Could you check a few things on this model? Use its own coordinates, in mm. A direction names the side the tool comes from. Round coordinates to 2 decimals unless told otherwise and drop trailing zeros. Write each loop counter-clockwise with the first axis right and the second up, starting at its lowest first coordinate (ties: lowest second). Pieces come first, ordered by that corner, then holes.
```python
from build123d import *

# Parameters (mm, degrees)
F0_R      = 37.5
F1_DEPTH  = 1
F2_R      = 36
F3_DEPTH  = 4
F4_R      = 37.5
F4_R_2    = 36
F5_DEPTH  = 1
F7_DEPTH  = 6
F8_DEPTH  = 1
F9_R      = 2.5
F10_DEPTH = 20


with BuildPart() as f1:
    # F0 (on Front) → F1 (new body)
    with BuildSketch(Plane.XZ):
        Circle(F0_R)
    extrude(amount=F1_DEPTH)

    # F2 (on face) → F3 (join)
    with BuildSketch(Plane.XZ.offset(1)):
        Circle(F2_R)
    extrude(amount=F3_DEPTH)

    # F4 (on face) → F5 (join)
    with BuildSketch(Plane.XZ.offset(5)):
        Circle(F4_R)
        Circle(F4_R_2, mode=Mode.SUBTRACT)
    extrude(amount=F5_DEPTH)

    # F6 (on face) → F7 (join)
    with BuildSketch(Plane.XZ.offset(5)):
        with BuildLine():
            ThreePointArc((-14.3973607657, 4.3698820625), (-13.2562102609, 2.7015956993), (-14.8554257168, 1.4655075997))
            ThreePointArc((-14.8554257168, 1.4655075997), (-16.4714294815, 0.0592412802), (-14.9737084003, -1.4723868378))
            ThreePointArc((-14.9737084003, -1.4723868378), (-13.2809972538, -2.5769830711), (-14.2854492449, -4.3309728264))
            ThreePointArc((-14.2854492449, -4.3309728264), (-15.2402872256, -6.2486113636), (-13.270444668, -7.0904981892))
            ThreePointArc((-13.270444668, -7.0904981892), (-13.2509857133, -7.078215185), (-13.2313372043, -7.0662377391))
            ThreePointArc((-13.2313372043, -7.0662377391), (-11.2704807141, -7.4819524915), (-11.5406426234, -9.4681019001))
            ThreePointArc((-11.5406426234, -9.4681019001), (-11.5683788085, -9.4914339833), (-11.5955323776, -9.515441602))
            ThreePointArc((-11.5955323776, -9.515441602), (-11.6640462748, -11.6315042777), (-9.5468760318, -11.6291454669))
            ThreePointArc((-9.5468760318, -11.6291454669), (-9.5335988041, -11.6103508311), (-9.5200295189, -11.5917659551))
            ThreePointArc((-9.5200295189, -11.5917659551), (-7.5493471931, -11.2254490142), (-7.0388777787, -13.163798288))
            ThreePointArc((-7.0388777787, -13.163798288), (-6.3580749762, -15.1949459127), (-4.3698820625, -14.3973607657))
            ThreePointArc((-4.3698820625, -14.3973607657), (-2.7015956993, -13.2562102609), (-1.4655075997, -14.8554257168))
            ThreePointArc((-1.4655075997, -14.8554257168), (-0.0592412802, -16.4714294815), (1.4723868378, -14.9737084003))
            ThreePointArc((1.4723868378, -14.9737084003), (2.5769830711, -13.2809972538), (4.3309728264, -14.2854492449))
            ThreePointArc((4.3309728264, -14.2854492449), (6.2486113636, -15.2402872256), (7.0904981892, -13.270444668))
            ThreePointArc((7.0904981892, -13.270444668), (7.4632395293, -11.2838728073), (9.4681019001, -11.5406426234))
            ThreePointArc((9.4681019001, -11.5406426234), (11.6051695712, -11.6889493932), (11.6291454669, -9.5468760318))
            ThreePointArc((11.6291454669, -9.5468760318), (11.2132854236, -7.5688810145), (13.163798288, -7.0388777787))
            ThreePointArc((13.163798288, -7.0388777787), (15.1949459127, -6.3580749762), (14.3973607657, -4.3698820625))
            ThreePointArc((14.3973607657, -4.3698820625), (13.2562102609, -2.7015956993), (14.8554257168, -1.4655075997))
            ThreePointArc((14.8554257168, -1.4655075997), (16.4714294815, -0.0592412802), (14.9737084003, 1.4723868378))
            ThreePointArc((14.9737084003, 1.4723868378), (13.2809972538, 2.5769830711), (14.2854492449, 4.3309728264))
            ThreePointArc((14.2854492449, 4.3309728264), (15.2402872256, 6.2486113636), (13.270444668, 7.0904981892))
            ThreePointArc((13.270444668, 7.0904981892), (11.2838728073, 7.4632395293), (11.5406426234, 9.4681019001))
            ThreePointArc((11.5406426234, 9.4681019001), (11.6889493932, 11.6051695712), (9.5468760318, 11.6291454669))
            ThreePointArc((9.5468760318, 11.6291454669), (7.5688810145, 11.2132854236), (7.0388777787, 13.163798288))
            ThreePointArc((7.0388777787, 13.163798288), (6.3580749762, 15.1949459127), (4.3698820625, 14.3973607657))
            ThreePointArc((4.3698820625, 14.3973607657), (2.7015956993, 13.2562102609), (1.4655075997, 14.8554257168))
            ThreePointArc((1.4655075997, 14.8554257168), (0.0592412802, 16.4714294815), (-1.4723868378, 14.9737084003))
            ThreePointArc((-1.4723868378, 14.9737084003), (-2.5769830711, 13.2809972538), (-4.3309728264, 14.2854492449))
            ThreePointArc((-4.3309728264, 14.2854492449), (-6.2486113636, 15.2402872256), (-7.0904981892, 13.270444668))
            ThreePointArc((-7.0904981892, 13.270444668), (-7.4632395293, 11.2838728073), (-9.4681019001, 11.5406426234))
            ThreePointArc((-9.4681019001, 11.5406426234), (-11.6051695712, 11.6889493932), (-11.6291454669, 9.5468760318))
            ThreePointArc((-11.6291454669, 9.5468760318), (-11.2132854236, 7.5688810145), (-13.163798288, 7.0388777787))
            ThreePointArc((-13.163798288, 7.0388777787), (-15.1949459127, 6.3580749762), (-14.3973607657, 4.3698820625))
        make_face()
    extrude(amount=F7_DEPTH)

    # F8 (add): a face of the model
    f8_faces = [f1.faces().sort_by_distance(p)[0] for p in [
        (-34.9817662351, -5, 0),
    ]]
    extrude(f8_faces, amount=F8_DEPTH)

    # F9 (on face) → F10 (cut)
    with BuildSketch(Plane.XZ.offset(11)):
        Circle(F9_R)
    extrude(amount=-F10_DEPTH, mode=Mode.SUBTRACT)


solid = f1.part
```
Q1. On a 3-axis mill with a long thin cutter (end or side, diameter ignored), from which of +Z, -Z, +X, -X, +Y, -Y can I reach the whole of each face in a straight line? I mean faces 4 (the cylindrical face through (-0.54, -5.58, -2.44)), 5 (the cylindrical face through (-4.686, -2.972, 35.694)). Say none if no direction works.
Q2. Imagine slicing it at B-B, the plane x = 0. Write out the boundary of the cut face in (y, z), then the cut area to 3 significant figures.
Q3. Imagine slicing it at A-A, the plane z = 0. Write out the boundary of the cut face in (x, y).
Q4. If I drill on L1, parallel to Y at x = -20, z = 30.5; L2, parallel to Z at x = 0, y = -5.5; L3, parallel to Z at x = 0, y = -2.5, over which ranges is the centre line in solid material (lowest first)?
Q5. We'd pull the mould along Y, two halves only. Please class faces 1 (the flat face through (-34, -5, 14)), 2 (the cylindrical face through (-4.88, -5.49, 37.18)), 3 (the flat face through (8, -6, -16)): pulls with the +Y half, pulls with the -Y half, needs draft (parallel to the pull), parting line crosses it, or undercut.
Q6. I'm going to push flat-ended pins straight in: pin 1 Ø1.5 at (y, z) = (-5, 18) entering from -X; pin 2 Ø6 at (y, z) = (-8, 14) entering from -X; pin 3 Ø1.5 at (y, z) = (-6, 11) entering from -X; pin 4 Ø6.5 at (x, z) = (0, 0) entering from +Y. Where does each tip first touch, or does it pass through?
Q7. Imagine slicing it at C-C, the plane y = -2.5. Write out the boundary of the cut face in (x, z).
Q8. Imagine slicing it at D-D, the plane x = -27. Write out the boundary of the cut face in (y, z).
Results found:
1. face 4: +Y, -Y
1. face 5: none
2. outline: (-11, -16.47) - (-6, -16.47) - (-6, -37.5) - (-5, -37.5) - (-5, -36) - (-1, -36) - (-1, -37.5) - (0, -37.5) - (0, -2.5) - (-11, -2.5) - close; (-11, 2.5) - (0, 2.5) - (0, 37.5) - (-1, 37.5) - (-1, 36) - (-5, 36) - (-5, 37.5) - (-6, 37.5) - (-6, 16.47) - (-11, 16.47) - close
2. area: 548 mm2
3. outline: (-37.5, -6) - (-16.47, -6) - (-16.47, -11) - (-2.5, -11) - (-2.5, 0) - (-37.5, 0) - (-37.5, -1) - (-36, -1) - (-36, -5) - (-37.5, -5) - close; (2.5, -11) - (16.47, -11) - (16.47, -6) - (37.5, -6) - (37.5, -5) - (36, -5) - (36, -1) - (37.5, -1) - (37.5, 0) - (2.5, 0) - close
4. L1: y = -6 to -5, -1 to 0
4. L2: z = -37.5 to -2.5, 2.5 to 37.5
4. L3: z = -36 to -2.5, 2.5 to 36
5. face 1: undercut
5. face 2: needs draft
5. face 3: pulls with the -Y half
6. pin 1: stops at x = -33.3
6. pin 2: stops at x = -35.61
6. pin 3: stops at x = -36.07
6. pin 4: stops at y = 0
7. outline: circle Ø72 at (0, 0); hole circle Ø5 at (0, 0)
8. outline: (-6, -26.02) - (-5, -26.02) - (-5, -23.81) - (-1, -23.81) - (-1, -26.02) - (0, -26.02) - (0, 26.02) - (-1, 26.02) - (-1, 23.81) - (-5, 23.81) - (-5, 26.02) - (-6, 26.02) - close
